Answer from the drawing. Dimensions are ordinates in mm from the lowest x, y and z of the part. A direction names the side the tool comes from. Give positions to 0.01 mm unless a question says otherwise; leave off trailing zeros. Loops run counter-clockwise (first coordinate to the right, second up) from the corner with the lowest first, then second, coordinate; pieces in that order, holes last.
Item 1: Section B-B, the plane x = 23.5 is taken. Give the vertices of the cut face in (y, z).
Item 2: A tool of negligible diameter and unlimited length cuts with its end or side. For the marked faces 5, 6 and 7, from which of +Z, -Z, +X, -X, +Y, -Y can it reach the whole face along a straight path? Write none if from no direction.
Item 3: Each of these flat-tipped pins is pushed along its axis until it touches: pin 1 Ø1.5 at (y, z) = (9, 118.5) entering from +X; pin 2 Ø5 at (x, y) = (52.5, 12.5) entering from +Z. Where does it stop, or does it pass through?
Item 4: The mould has two halves that part along Z. Classify the marked faces 1, 2, 3 and 4: pulls with the +Z half, pulls with the -Z half, needs draft (parallel to the pull), parting line crosses it, or undercut.
Item 5: Section D-D, the plane x = 53 is taken. Give the vertices of the cut face in (y, z), and give its area (3 significant figures).
Item 6: Section C-C, the plane y = 17.25 is taken. Give the vertices of the cut face in (x, z).
Item 7: Consider line 1 along Z through (x, y) = (52, 8); line 2 along Z through (x, y) = (23, 9.75); line 3 along Z through (x, y) = (41.5, 13). Determine where each line is inside the solid, lowest interval first.
Item 8: Section A-A, the plane z = 93.5 is taken. Give the vertices of the cut face in (x, y), and give its area (3 significant figures).
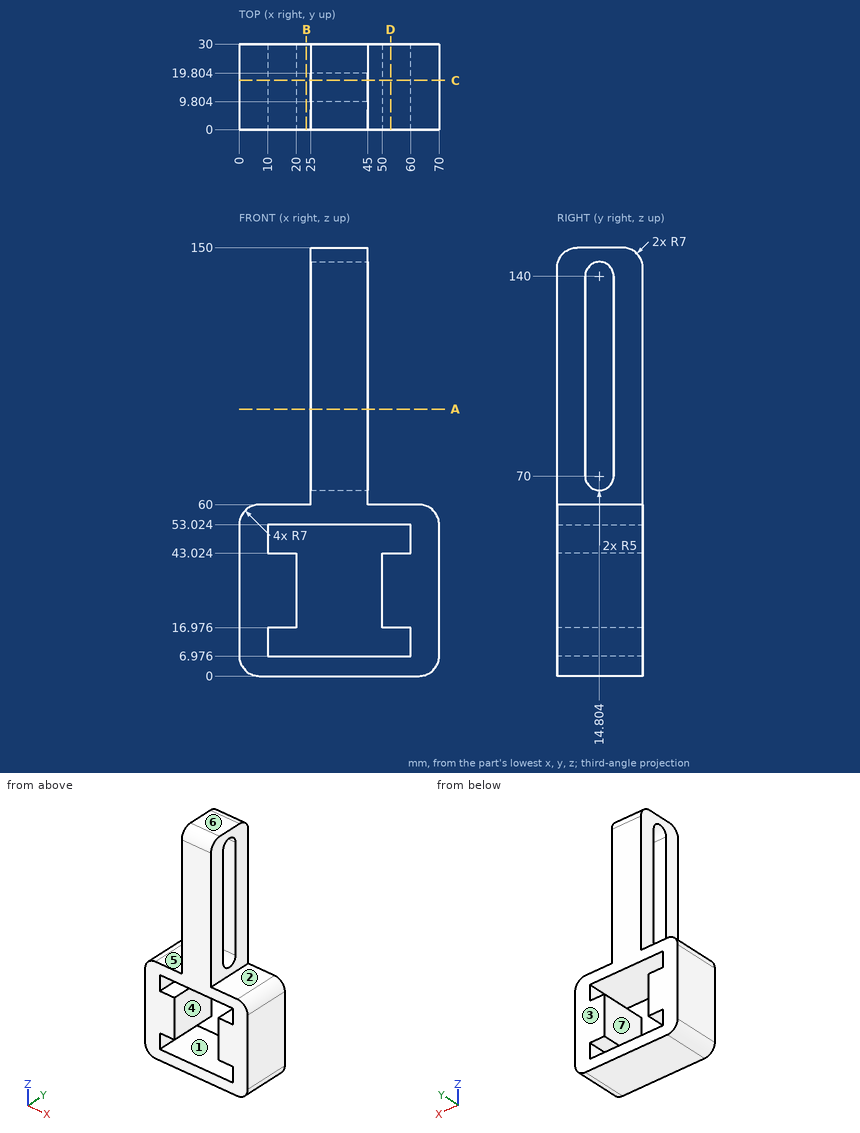
Worked answers:
1. outline: (0, 0) - (30, 0) - (30, 6.98) - (0, 6.98) - close; (0, 53.02) - (30, 53.02) - (30, 60) - (0, 60) - close
2. face 5: +Z, -X, +Y, -Y
2. face 6: +Z, +X, -X, +Y, -Y
2. face 7: +Y, -Y
3. pin 1: stops at x = 45
3. pin 2: stops at z = 60
4. face 1: undercut
4. face 2: pulls with the +Z half
4. face 3: needs draft
4. face 4: undercut
5. outline: (0, 0) - (30, 0) - (30, 6.98) - (0, 6.98) - close; (0, 16.98) - (30, 16.98) - (30, 43.02) - (0, 43.02) - close; (0, 53.02) - (30, 53.02) - (30, 60) - (0, 60) - close
5. area: 1,200 mm2
6. outline: (0, 7) arc R7 ccw to (7, 0) - (63, 0) arc R7 ccw to (70, 7) - (70, 53) arc R7 ccw to (63, 60) - (45, 60) - (45, 65.64) - (25, 65.64) - (25, 60) - (7, 60) arc R7 ccw to (0, 53) - close; (25, 144.36) - (45, 144.36) - (45, 150) - (25, 150) - close; hole (10, 6.98) - (60, 6.98) - (60, 16.98) - (50, 16.98) - (50, 43.02) - (60, 43.02) - (60, 53.02) - (10, 53.02) - (10, 43.02) - (20, 43.02) - (20, 16.98) - (10, 16.98) - close
7. line 1: z = 0 to 6.98, 16.98 to 43.02, 53.02 to 60
7. line 2: z = 0 to 6.98, 53.02 to 60
7. line 3: z = 0 to 6.98, 53.02 to 65.34, 144.66 to 150
8. outline: (25, 0) - (45, 0) - (45, 9.8) - (25, 9.8) - close; (25, 19.8) - (45, 19.8) - (45, 30) - (25, 30) - close
8. area: 400 mm2
